from build123d import *

# Parameters (mm, degrees)
SKETCH1_R            = 8.75
BOSS_EXTRUDE1_DEPTH  = 6
SKETCH2_R            = 8.25
SKETCH2_R_2          = 3.75
CUT_EXTRUDE1_DEPTH   = 5
SKETCH3_R            = 2.5
CUT_EXTRUDE2_DEPTH   = 20
BOSS_EXTRUDE3_START  = 1
SKETCH5_R            = 3.75
SKETCH5_R_2          = 2.5
BOSS_EXTRUDE3_DEPTH  = 1
SKETCH4_R            = 6.25
BOSS_EXTRUDE4_DEPTH  = 2
SKETCH7_R            = 8.75
BOSS_EXTRUDE5_DEPTH  = 2
SKETCH9_R            = 6.25
BOSS_EXTRUDE6_DEPTH  = 2
SKETCH10_R           = 8.75
BOSS_EXTRUDE7_DEPTH  = 2
SKETCH11_R           = 2.5
CUT_EXTRUDE4_DEPTH   = 15.735162028
SKETCH12_R           = 3.1
BOSS_EXTRUDE8_DEPTH  = 1
SKETCH13_R           = 3.065
CUT_EXTRUDE5_DEPTH   = 1
CUT_EXTRUDE6_START   = -1
SKETCH15_R           = 8.25
CUT_EXTRUDE6_DEPTH   = 1
SKETCH16_R           = 3.15
SKETCH16_R_2         = 2.85
BOSS_EXTRUDE10_DEPTH = 2
BOSS_EXTRUDE11_DEPTH = 1
CIRPATTERN1_START    = 14
CIRPATTERN1_DEPTH    = 1


# Read off the part's stored shape, not the designer's step: CirPattern1
with BuildPart() as part:
    # Sketch1 → Boss-Extrude1 (new body)
    with BuildSketch(Plane(origin=(0, 0, 0), x_dir=(1, 0, 0), z_dir=(0, 1, 0))):
        with Locations(Location((0, 0, 0), (0, 0, 270))):
            Circle(SKETCH1_R)
    extrude(amount=BOSS_EXTRUDE1_DEPTH)

    # Sketch2 → Cut-Extrude1 (cut)
    with BuildSketch(Plane.XZ):
        with Locations(Location((0, 0, 0), (0, 0, 270))):
            Circle(SKETCH2_R)
        with Locations(Location((0, 0, 0), (0, 0, 270))):
            Circle(SKETCH2_R_2, mode=Mode.SUBTRACT)
    extrude(amount=-CUT_EXTRUDE1_DEPTH, mode=Mode.SUBTRACT)

    # Sketch3 → Cut-Extrude2 (cut)
    with BuildSketch(Plane.XZ):
        with Locations(Location((0, 0, 0), (0, 0, 270))):
            Circle(SKETCH3_R)
    extrude(amount=-CUT_EXTRUDE2_DEPTH, mode=Mode.SUBTRACT)

    # Sketch5 → Boss-Extrude3 (add)
    with BuildSketch(Plane.XZ.offset(BOSS_EXTRUDE3_START)):
        with Locations(Location((0, 0, 0), (0, 0, 270))):
            Circle(SKETCH5_R)
        with Locations(Location((0, 0, 0), (0, 0, 270))):
            Circle(SKETCH5_R_2, mode=Mode.SUBTRACT)
    extrude(amount=-BOSS_EXTRUDE3_DEPTH)

    # Sketch4 → Boss-Extrude4 (add)
    with BuildSketch(Plane(origin=(0, 6, 0), x_dir=(1, 0, 0), z_dir=(0, 1, 0))):
        with Locations(Location((0, 0, 0), (0, 0, 270))):
            Circle(SKETCH4_R)
    extrude(amount=BOSS_EXTRUDE4_DEPTH)

    # Sketch7 → Boss-Extrude5 (add)
    with BuildSketch(Plane(origin=(0, 8, 0), x_dir=(1, 0, 0), z_dir=(0, 1, 0))):
        with Locations(Location((0, 0, 0), (0, 0, 270))):
            Circle(SKETCH7_R)
    extrude(amount=BOSS_EXTRUDE5_DEPTH)

    # Sketch9 → Boss-Extrude6 (add)
    with BuildSketch(Plane(origin=(0, 10, 0), x_dir=(1, 0, 0), z_dir=(0, 1, 0))):
        with Locations(Location((0, 0, 0), (0, 0, 270))):
            Circle(SKETCH9_R)
    extrude(amount=BOSS_EXTRUDE6_DEPTH)

    # Sketch10 → Boss-Extrude7 (add)
    with BuildSketch(Plane(origin=(0, 12, 0), x_dir=(1, 0, 0), z_dir=(0, 1, 0))):
        with Locations(Location((0, 0, 0), (0, 0, 270))):
            Circle(SKETCH10_R)
    extrude(amount=BOSS_EXTRUDE7_DEPTH)

    # Sketch11 → Cut-Extrude4 (cut, through all)
    with BuildSketch(Plane.XZ.offset(-6)):
        with Locations(Location((0, 0, 0), (0, 0, 270))):
            Circle(SKETCH11_R)
    extrude(amount=-CUT_EXTRUDE4_DEPTH, mode=Mode.SUBTRACT)

    # Sketch12 → Boss-Extrude8 (add)
    with BuildSketch(Plane(origin=(0, 14, 0), x_dir=(1, 0, 0), z_dir=(0, 1, 0))):
        with Locations(Location((0, 0, 0), (0, 0, 270))):
            Circle(SKETCH12_R)
    extrude(amount=BOSS_EXTRUDE8_DEPTH)

    # Sketch13 → Cut-Extrude5 (cut)
    with BuildSketch(Plane(origin=(0, 15, 0), x_dir=(1, 0, 0), z_dir=(0, 1, 0))):
        with Locations(Location((0, 0, 0), (0, 0, 270))):
            Circle(SKETCH13_R)
    extrude(amount=-CUT_EXTRUDE5_DEPTH, mode=Mode.SUBTRACT)

    # Sketch15 → Cut-Extrude6 (cut)
    with BuildSketch(Plane(origin=(0, 15, 0), x_dir=(1, 0, 0), z_dir=(0, 1, 0)).offset(CUT_EXTRUDE6_START)):
        with Locations(Location((0, 0, 0), (0, 0, 90))):
            Circle(SKETCH15_R)
    extrude(amount=CUT_EXTRUDE6_DEPTH, mode=Mode.SUBTRACT)

    # Sketch16 → Boss-Extrude10 (add)
    with BuildSketch(Plane(origin=(0, 14, 0), x_dir=(1, 0, 0), z_dir=(0, 1, 0))):
        with Locations(Location((0, 0, 0), (0, 0, 270))):
            Circle(SKETCH16_R)
        with Locations(Location((0, 0, 0), (0, 0, 270))):
            Circle(SKETCH16_R_2, mode=Mode.SUBTRACT)
    extrude(amount=BOSS_EXTRUDE10_DEPTH)

    # Sketch14 → Boss-Extrude11 (add)
    with BuildSketch(Plane(origin=(0, 14, 0), x_dir=(1, 0, 0), z_dir=(0, 1, 0))):
        Polygon((0.998161763, 8.189393939), (0.684499773, 3.023484755), (1.533676009, 2.694037472), (1.858150244, 8.038020756), align=None)
    extrude(amount=BOSS_EXTRUDE11_DEPTH)

    # CirPattern1 outline → CirPattern1 (add)
    with BuildSketch(Plane(origin=(0, 0, 0), x_dir=(1, 0, 0), z_dir=(0, 1, 0)).offset(CIRPATTERN1_START)):
        with BuildLine():
            Line((-6.324565807, 5.297392505), (-2.203633173, 2.2508889))
            ThreePointArc((-2.203633173, 2.2508889), (-1.85566188, 2.545391716), (-1.468825776, 2.786584081))
            Line((-1.468825776, 2.786584081), (-5.729230277, 5.936195788))
            Line((-5.729230277, 5.936195788), (-6.324565807, 5.297392505))
        make_face()
        with BuildLine():
            ThreePointArc((-3.129074903, 0.362477928), (-3.043987046, 0.810335032), (-2.895146203, 1.241220553))
            Line((-2.895146203, 1.241220553), (-8.188217227, 1.007769145))
            Line((-8.188217227, 1.007769145), (-8.248867898, 0.136668965))
            Line((-8.248867898, 0.136668965), (-3.129074903, 0.362477928))
        make_face()
        with BuildLine():
            Line((-4.378035213, 6.992517978), (-1.400216766, 2.821682656))
            ThreePointArc((-1.400216766, 2.821682656), (-0.978270026, 2.994242435), (-0.535834488, 3.104091075))
            Line((-0.535834488, 3.104091075), (-3.614436407, 7.416087207))
            Line((-3.614436407, 7.416087207), (-4.378035213, 6.992517978))
        make_face()
        with BuildLine():
            ThreePointArc((-3.087938917, -0.622200326), (-3.145411012, -0.169969315), (-3.137005907, 0.285821517))
            Line((-3.137005907, 0.285821517), (-8.098875142, -1.571852864))
            Line((-8.098875142, -1.571852864), (-7.887372599, -2.419060455))
            Line((-7.887372599, -2.419060455), (-3.087938917, -0.622200326))
        make_face()
        with BuildLine():
            Line((3.47997015, 7.480127523), (1.603849487, 2.711119109))
            ThreePointArc((1.603849487, 2.711119109), (1.97837896, 2.451227588), (2.311473446, 2.139997782))
            Line((2.311473446, 2.139997782), (4.251090913, 7.070412014))
            Line((4.251090913, 7.070412014), (3.47997015, 7.480127523))
        make_face()
        with BuildLine():
            ThreePointArc((-2.008215906, -2.426843397), (-2.337478309, -2.111562255), (-2.61778478, -1.752056747))
            Line((-2.61778478, -1.752056747), (-5.30480905, -6.318346377))
            Line((-5.30480905, -6.318346377), (-4.60727569, -6.843647471))
            Line((-4.60727569, -6.843647471), (-2.008215906, -2.426843397))
        make_face()
        with BuildLine():
            Line((8.168690382, 1.155420894), (3.14725484, 0.131479935))
            ThreePointArc((3.14725484, 0.131479935), (3.133274841, -0.324173978), (3.053671823, -0.773038421))
            Line((3.053671823, -0.773038421), (8.245056512, 0.285557547))
            Line((8.245056512, 0.285557547), (8.168690382, 1.155420894))
        make_face()
        with BuildLine():
            ThreePointArc((-1.159990971, -2.92863807), (-1.570565356, -2.730535563), (-1.948245964, -2.47524497))
            Line((-1.948245964, -2.47524497), (-3.092696808, -7.648380643))
            Line((-3.092696808, -7.648380643), (-2.266976195, -7.932422009))
            Line((-2.266976195, -7.932422009), (-1.159990971, -2.92863807))
        make_face()
        with BuildLine():
            Line((8.125930909, -1.42539358), (3.033846758, -0.847510382))
            ThreePointArc((3.033846758, -0.847510382), (2.879746187, -1.276542948), (2.665332476, -1.678839716))
            Line((2.665332476, -1.678839716), (7.929756858, -2.276281216))
            Line((7.929756858, -2.276281216), (8.125930909, -1.42539358))
        make_face()
        with BuildLine():
            ThreePointArc((0.941569357, -3.00598522), (0.497823185, -3.11041349), (0.04365065, -3.149697544))
            Line((0.04365065, -3.149697544), (2.409805062, -7.890205293))
            Line((2.409805062, -7.890205293), (3.230263526, -7.591304075))
            Line((3.230263526, -7.591304075), (0.941569357, -3.00598522))
        make_face()
        with BuildLine():
            Line((5.418005144, -6.221552882), (1.824386191, -2.567900899))
            ThreePointArc((1.824386191, -2.567900899), (1.434628612, -2.804343193), (1.014824303, -2.982051581))
            Line((1.014824303, -2.982051581), (4.730068332, -6.759360441))
            Line((4.730068332, -6.759360441), (5.418005144, -6.221552882))
        make_face()
    extrude(amount=CIRPATTERN1_DEPTH)


solid = part.part
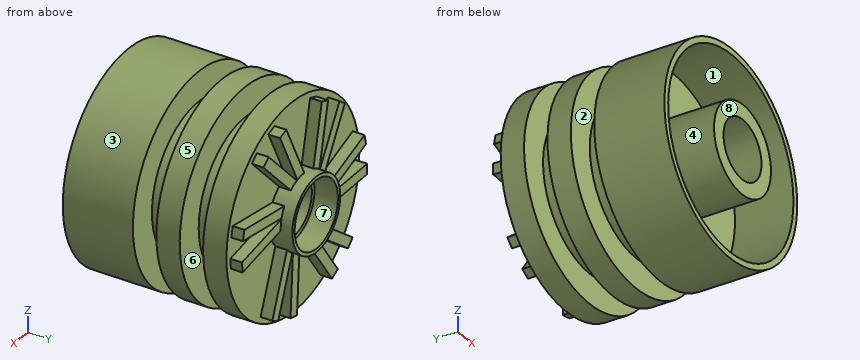
Here's how the part is built. I have some questions about the finished solid (model axes, mm). Face numbers are marked on the shaded views. A direction names the side the tool comes from. Round coordinates to 2 decimals unless told otherwise and drop trailing zeros. Order: outer loops, then holes, each group sorted by start corner. A loop starts at its lowest first (then second) coordinate and runs counter-clockwise, first axis right, second up. Notation, with made-up numbers: M -22,65.25 L 7,65.25 A36 ccw 7,99.25 Z; hole C 42.25,7 d5. An arc over 180 degrees is marked long. Return JSON: item names as keys, results as strings. Group by question number.
1. If we section it at A-A on y = 6.75: List the corners of the cut face in (x, z) for me, then the cut area to 3 significant figures.
2. Please list where these lines run through material, in increasing order: probe 1 along Y at (x, z) = (2.75, 6.5); probe 2 along X at (y, z) = (3.8, 0); probe 3 along Y at (x, z) = (2, 7).
3. On a 3-axis mill with a long thin cutter (end or side, diameter ignored), from which of +Z, -Z, +X, -X, +Y, -Y can I reach the whole of each face in a straight line? I mean the marked faces 4, 5, 6, 7 and 8. Say none if no direction works.
4. If we mould it in two halves opening along Z, with no side actions, what happens to the marked faces 1, 2 and 3? For each: pulls with the +Z half, pulls with the -Z half, needs draft (parallel to the pull), parting line crosses it, or undercut.
5. If we section it at B-B on y = 12.25: List the corners of the cut face in (x, z) for me.
6. I'm going to push flat-ended pins straight in: pin 1 Ø2 at (x, z) = (-5.5, -3) entering from +Y; pin 2 Ø3 at (x, y) = (7, 10.5) entering from -Z; pin 3 Ø8 at (y, z) = (3, 5.5) entering from -X. Where does each tip first touch, or does it pass through?
Reply:
{
 "1": {"outline": "C 0,0 d12.5; hole C 0,0 d5", "area": "103 mm^2"},
 "2": {"probe 1": "5 to 6, 8 to 10, 12 to 14", "probe 2": "-8.75 to -8.25, -3.75 to -2.5, 2.5 to 3.75, 8.25 to 8.75", "probe 3": "5 to 6, 8 to 10, 12 to 15"},
 "3": {"face 4": "-Y", "face 5": "+Y, -Y", "face 6": "none", "face 7": "+Y", "face 8": "+Z, -Z, +X, -X, -Y"},
 "4": {"face 1": "undercut", "face 2": "needs draft", "face 3": "parting line crosses it"},
 "5": {"outline": "C 0,0 d17.5; hole C 0,0 d5"},
 "6": {"pin 1": "y = 14", "pin 2": "z = -6.74", "pin 3": "x = -8.62"}
}
